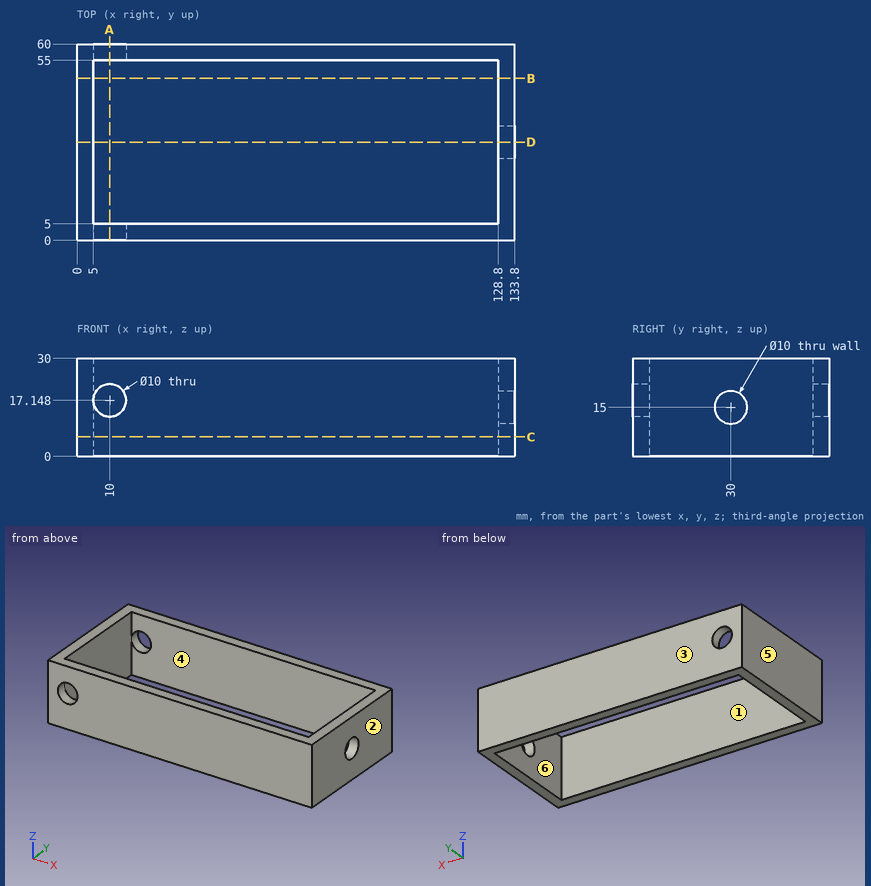
Can you work these out from the drawing? Everything is in mm from the part's minimum corner. A direction names the side the tool comes from. Give positions to 0.01 mm unless a question says otherwise; leave off trailing zeros. Order: outer loops, then holes, each group sorted by start corner. A loop starts at its lowest first (then second) coordinate and runs counter-clockwise, first axis right, second up.
1. Suppose I cut it at A-A (x = 10). List the corners of the cut face in (y, z) for me.
2. We'd pull the mould along X, two halves only. Please class the marked faces 3, 4, 5 and 6: pulls with the +X half, pulls with the -X half, needs draft (parallel to the pull), parting line crosses it, or undercut.
3. For the marked faces 1 and 2, which set-ups out of +Z, -Z, +X, -X, +Y, -Y let a thin tool reach every point of the face, with its end or its side?
4. Suppose I cut it at D-D (y = 30). List the corners of the cut face in (x, z) for me.
5. Suppose I cut it at B-B (y = 49.5). List the corners of the cut face in (x, z) for me.
6. Suppose I cut it at C-C (z = 6). List the corners of the cut face in (x, y) for me.
7. I need wall thicknesses on L1, parallel to X at y = 10, z = 19; L2, parallel to Y at x = 120.5, z = 16; L3, parallel to Y at x = 130.6, z = 15. Which ranges of each line are inside material? Lowest first, please.
Solved:
1. outline: (0, 0) - (5, 0) - (5, 12.15) - (0, 12.15) - close; (0, 22.15) - (5, 22.15) - (5, 30) - (0, 30) - close; (55, 0) - (60, 0) - (60, 12.15) - (55, 12.15) - close; (55, 22.15) - (60, 22.15) - (60, 30) - (55, 30) - close
2. face 3: needs draft
2. face 4: undercut
2. face 5: pulls with the -X half
2. face 6: undercut
3. face 1: +Z, -Z
3. face 2: +Z, -Z, +X, +Y, -Y
4. outline: (0, 0) - (5, 0) - (5, 30) - (0, 30) - close; (128.8, 0) - (133.8, 0) - (133.8, 10) - (128.8, 10) - close; (128.8, 20) - (133.8, 20) - (133.8, 30) - (128.8, 30) - close
5. outline: (0, 0) - (5, 0) - (5, 30) - (0, 30) - close; (128.8, 0) - (133.8, 0) - (133.8, 30) - (128.8, 30) - close
6. outline: (0, 0) - (133.8, 0) - (133.8, 60) - (0, 60) - close; hole (5, 5) - (128.8, 5) - (128.8, 55) - (5, 55) - close
7. L1: x = 0 to 5, 128.8 to 133.8
7. L2: y = 0 to 5, 55 to 60
7. L3: y = 0 to 25, 35 to 60
